Input: part model. Units: mm. Frame: model coordinates. A direction names the side the tool comes from. Round coordinates to 2 decimals unless told otherwise and drop trailing zeros. Order: outer loops, then holes, each group sorted by start corner. A loop starts at its lowest first (then second) coordinate and runs counter-clockwise, first axis right, second up.
Item 1: Cut plane A-A on x = -2.25. Output: boundary loops of the cut face in (y, z), then the cut area to 3 significant figures.
Item 2: Mould query, pull axis Y, two halves, no side actions, for faces 1 (the flat face through (0, -3.5, -3)), 2 (the flat face through (-0.348, 0.793, -0.886)), 3 (the flat face through (1, 0, 0.1)). Classes: released by +Y, released by -Y, zero draft, split by the parting line, or undercut.
Item 3: Cut plane B-B on y = 3.25. Output: boundary loops of the cut face in (x, z), then the cut area to 3 significant figures.
Item 4: Line query: L1, parallel to X at y = 2.25, z = -1.75; L2, parallel to Z at x = -2.25, y = 0; L3, parallel to Z at x = 1.75, y = 3. Output: solid intervals per line, ascending.
Item 5: Reachability of faces 4 (the flat face through (-2.88, 3.01, -1.88)), 5 (the flat face through (0, 0, -1.9)), 6 (the flat face through (0, 3, -1.25)), 7 (the flat face through (3.13, 1.44, -1.23)), 8 (the flat face through (-3.145, 1.424, -1.232)) from +Z, -Z, +X, -X, +Y, -Y: full face, straight path, thin tool, end or side. Return the list, or none.
Item 6: First-contact query: pin 1 (0.6 mm diameter, centred on x = 2, y = 1.5, fed in from +Z); pin 2 (0.5 mm diameter, centred on x = -0.5, y = 3, fed in from +Z). Flat tips, straight axial feed; report the tip coordinate or a pass-through.
```python
from build123d import *

# Parameters (mm, degrees)
BASE_EXTRUDE_START  = -6
SKETCH1_W           = 7
SKETCH1_H           = 7
BASE_EXTRUDE_DEPTH  = 6
SKETCH2_R           = 1.5
CUT_EXTRUDE1_DEPTH  = 3
SKETCH3_R           = 1.48
BOSS_EXTRUDE1_DEPTH = 3.1
CUT_EXTRUDE2_DEPTH  = 2
CUT_EXTRUDE3_DEPTH  = 0.5
CUT_EXTRUDE4_DEPTH  = 2.5
BOSS_EXTRUDE2_DEPTH = 1.25


with BuildPart() as part:
    # Sketch1 → Base-Extrude (new body)
    with BuildSketch(Plane.XY.offset(BASE_EXTRUDE_START)):
        Rectangle(SKETCH1_W, SKETCH1_H)
    extrude(amount=BASE_EXTRUDE_DEPTH)

    # Sketch2 → Cut-Extrude1 (cut)
    with BuildSketch(Plane.XY):
        Circle(SKETCH2_R)
    extrude(amount=-CUT_EXTRUDE1_DEPTH, mode=Mode.SUBTRACT)

    # Sketch3 → Boss-Extrude1 (add)
    with BuildSketch(Plane.XY.offset(-3)):
        Circle(SKETCH3_R)
    extrude(amount=BOSS_EXTRUDE1_DEPTH)

    # Sketch4 → Cut-Extrude2 (cut)
    with BuildSketch(Plane.XY.offset(0.1)):
        with BuildLine():
            Line((0.724096874, -1.290768654), (-0.039924426, -0.279012083))
            Line((-0.039924426, -0.279012083), (-0.743721804, -0.81048003))
            ThreePointArc((-0.743721804, -0.81048003), (-0.87868568, -0.661748801), (-0.984357933, -0.490957696))
            Line((-0.984357933, -0.490957696), (-0.280973901, 0.040198115))
            Line((-0.280973901, 0.040198115), (-1.043307072, 1.049719178))
            ThreePointArc((-1.043307072, 1.049719178), (-0.891883058, 1.181077733), (-0.724096874, 1.290768654))
            Line((-0.724096874, 1.290768654), (0.038236297, 0.28124759))
            Line((0.038236297, 0.28124759), (0.741620329, 0.812403402))
            ThreePointArc((0.741620329, 0.812403402), (0.876968937, 0.664022201), (0.98308315, 0.493505339))
            Line((0.98308315, 0.493505339), (0.279285772, -0.037962608))
            Line((0.279285772, -0.037962608), (1.043307072, -1.049719178))
            ThreePointArc((1.043307072, -1.049719178), (0.891883058, -1.181077733), (0.724096874, -1.290768654))
        make_face()
    extrude(amount=-CUT_EXTRUDE2_DEPTH, mode=Mode.SUBTRACT)

    # Sketch5 → Cut-Extrude3 (cut)
    with BuildSketch(Plane.XY):
        Polygon((1.3, 1.2), (1.931123884, 1.691612289), (2.115478493, 1.454940832), (1.484354608, 0.963328543), align=None)
        Polygon((1.689974186, 0.523437915), (2.471261862, 0.695454097), (2.53576793, 0.402471219), (1.754480254, 0.230455037), align=None)
        Polygon((1.750691662, -0.255105281), (2.529925297, -0.436199021), (2.462015144, -0.728411634), (1.68278151, -0.547317894), align=None)
        Polygon((1.470322877, -0.98394646), (2.095684825, -1.482867731), (1.908589348, -1.717378462), (1.283227401, -1.21845719), align=None)
        Polygon((0.903491923, -1.52108591), (1.25314327, -2.240630165), (0.983314174, -2.371749421), (0.633662827, -1.652205165), align=None)
        Polygon((0.160634151, -1.761873057), (0.166452524, -2.561851898), (-0.133539541, -2.564033789), (-0.139357915, -1.764054947), align=None)
        Polygon((-0.613519882, -1.659395479), (-0.952668072, -2.383949483), (-1.224375823, -2.256768912), (-0.885227633, -1.532214907), align=None)
        Polygon((-1.268142184, -1.233618823), (-1.886180889, -1.741583546), (-2.07666766, -1.509819032), (-1.458628956, -1.001854309), align=None)
        Polygon((-1.675693067, -0.567496913), (-2.452210156, -0.759905877), (-2.524363518, -0.468711968), (-1.747846428, -0.276303004), align=None)
        Polygon((-1.756769622, 0.209190097), (-2.540476714, 0.369823822), (-2.480239067, 0.663713982), (-1.696531975, 0.503080257), align=None)
        Polygon((-1.49557575, 0.94512072), (-2.133783638, 1.427500956), (-1.952891049, 1.666828914), (-1.314683162, 1.184448678), align=None)
    extrude(amount=-CUT_EXTRUDE3_DEPTH, mode=Mode.SUBTRACT)

    # Sketch7 → Cut-Extrude4 (cut)
    with BuildSketch(Plane.XY):
        Polygon((3.5, 3.5), (-3.5, 3.5), (-3.5, 1), (-2.779166508, 1.859055904), (-3.066312501, 2.1), (-3.066312501, 2.5), (3.066312501, 2.5), (3.066312501, 2.1), (2.779166508, 1.859055904), (3.5, 1), align=None)
    extrude(amount=-CUT_EXTRUDE4_DEPTH, mode=Mode.SUBTRACT)

    # Sketch8 → Boss-Extrude2 (add)
    with BuildSketch(Plane.XY.offset(-2.5)):
        Polygon((-3.066312501, 2.5), (3.066312501, 2.5), (2.70444426, 3.5), (-2.70444426, 3.5), align=None)
    extrude(amount=BOSS_EXTRUDE2_DEPTH)


solid = part.part
```
From the geometry:
1. outline: (-3.5, -6) - (3.5, -6) - (3.5, -1.25) - (2.5, -1.25) - (2.5, 0) - (0.62, 0) - (0.62, -0.5) - (0.31, -0.5) - (0.31, 0) - (-0.4, 0) - (-0.4, -0.5) - (-0.71, -0.5) - (-0.71, 0) - (-3.5, 0) - close
1. area: 40.4 mm2
2. face 1: released by -Y
2. face 2: undercut
2. face 3: zero draft
3. outline: (-3.5, -6) - (3.5, -6) - (3.5, -2.5) - (2.79, -2.5) - (2.79, -1.25) - (-2.79, -1.25) - (-2.79, -2.5) - (-3.5, -2.5) - close
3. area: 31.5 mm2
4. L1: x = -3.07 to 3.07
4. L2: z = -6 to 0
4. L3: z = -6 to -1.25
5. face 4: +Z, -X, +Y
5. face 5: +Z
5. face 6: +Z, +X, -X, +Y
5. face 7: +Z, +X
5. face 8: +Z, -X
6. pin 1: stops at z = 0
6. pin 2: stops at z = -1.25
